For this review, use the dimensioned drawing (mm, ordinates from the lowest corner) and the shaded views. Coordinates: 2 decimals unless noted, no trailing zeros. Order: outer loops, then holes, each group sorted by start corner. A loop starts at its lowest first (then second) coordinate and runs counter-clockwise, first axis right, second up. Notation, with made-up numbers: (53, 31) -> (83, 31) arc R5 cw to (83, 40) -> close; hole circle Ø11 at (31, 64). An arc over 180 degrees is marked (long way). Return JSON: item names as keys, results as strings. Group by question number.
Item 1: Take a section at A-A (x = 5). Write out the cut boundary in (y, z), then the cut area to 3 significant figures.
Item 2: For line 1 along Z through (x, y) = (6.5, 4.5) (1 decimal); line 2 along Z through (x, y) = (3.25, 2.25); line 3 along Y through (x, z) = (4, 14.5), list the stretches that pass through material, from the lowest coordinate up.
Item 3: Take a section at B-B (y = 7). Write out the cut boundary in (x, z).
Item 4: Take a section at D-D (x = 7.5). Write out the cut boundary in (y, z).
Item 5: Draft analysis for pull direction Z (two halves, no side actions). For the marked faces 1, 2 and 3, state which applies: +Z half, -Z half, draft (parallel to the pull), parting line (faces both ways), or undercut.
Item 6: Insertion check: pin 1 (1 mm diameter, centred on x = 5.5, y = 6.5, fed in from -Z); pin 2 (1 mm diameter, centred on y = 2.5, z = 27.5, fed in from -X); pin 3 (1.5 mm diameter, centred on x = 4, z = 19.5, fed in from +Y). Each pin has a flat end and moves straight along its axis. Give the tip position at first contact, or say it passes through.
Item 7: Take a section at C-C (z = 3). Write out the cut boundary in (x, y).
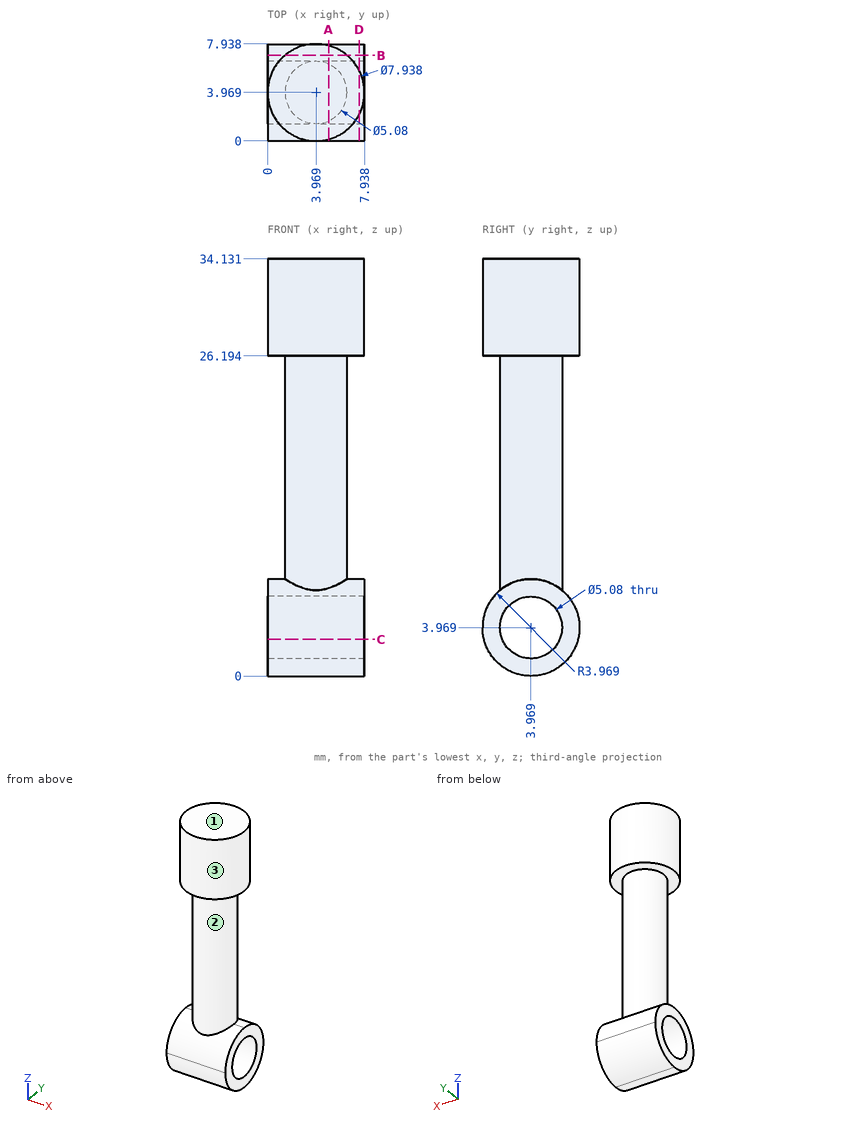
Findings below:
{
 "1": {"outline": "(0.14, 26.19) -> (1.65, 26.19) -> (1.65, 7.19) arc R3.97 ccw (long way) to (6.29, 7.19) -> (6.29, 26.19) -> (7.8, 26.19) -> (7.8, 34.13) -> (0.14, 34.13) -> close; hole circle Ø5.08 at (3.97, 3.97)", "area": "176 mm2"},
 "2": {"line 1": "z = 0 to 1.5, 6.5 to 7.9, 26.2 to 34.1", "line 2": "z = 0.39 to 2.1, 5.84 to 34.13", "line 3": "y = 1.43 to 6.51"},
 "3": {"outline": "(0, 1.41) -> (7.94, 1.41) -> (7.94, 6.53) -> (0, 6.53) -> close; (1.41, 26.19) -> (6.53, 26.19) -> (6.53, 34.13) -> (1.41, 34.13) -> close"},
 "4": {"outline": "circle Ø7.94 at (3.97, 3.97); (2.16, 26.19) -> (5.78, 26.19) -> (5.78, 34.13) -> (2.16, 34.13) -> close; hole circle Ø5.08 at (3.97, 3.97)"},
 "5": {"face 1": "+Z half", "face 2": "undercut", "face 3": "draft"},
 "6": {"pin 1": "stops at z = 0.56", "pin 2": "stops at x = 0.12", "pin 3": "stops at y = 6.51"},
 "7": {"outline": "(0, 0.12) -> (7.94, 0.12) -> (7.94, 1.62) -> (0, 1.62) -> close; (0, 6.32) -> (7.94, 6.32) -> (7.94, 7.82) -> (0, 7.82) -> close"}
}
